Read the model definition and answer for the solid it produces. Units are mm, in the model's axes. Coordinates: 2 decimals unless noted, no trailing zeros. Write each loop counter-clockwise with the first axis right and the second up, starting at its lowest first coordinate (ties: lowest second). Pieces come first, ordered by that corner, then holes.
(1) Section A-A on x = 0.35 is taken. State how many separate pieces and enclosed holes the cut face has, then the cut area to 3 significant figures.
(2) Find the intervals of material crossed by probe 1 along Z at (x, y) = (0.4, 275); probe 2 along Y at (x, z) = (0.95, -1); probe 3 along Z at (x, y) = (0.7, 263.5), in increasing order.
(3) Section C-C on z = -7.5 is taken. Write down the section's boundary in (x, y).
(4) Given pin 1 (12 mm diameter, centred on y = 94.5, z = -6, fed in from -X); pin 2 (0.5 mm diameter, centred on x = 0.5, z = 15.5, fed in from +Y); pin 3 (0.5 mm diameter, centred on x = 0.5, z = 23, fed in from -Y), each flat-ended and moving along its own axis, determine where each tip first touches the part or whether it passes through.
from build123d import *

# Parameters (mm, degrees)
F1_DEPTH = 1


with BuildPart() as f1:
    # F0 (on Right) → F1 (new body)
    with BuildSketch(Plane.YZ):
        Polygon((289.166, 39.710689), (-29.834, 39.710689), (-56.334, 39.710689), (-56.334, 32.210689), (-29.834, 32.210689), (-29.834, -16.289311), (289.166, -16.289311), (289.166, 32.210689), (315.666, 32.210689), (315.666, 39.710689), align=None)
        with BuildLine():
            ThreePointArc((-24.167, 27.710689), (-23.581214, 29.124903), (-22.167, 29.710689))
            Line((-22.167, 29.710689), (-13.167, 29.710689))
            ThreePointArc((-13.167, 29.710689), (-11.752786, 29.124903), (-11.167, 27.710689))
            Line((-11.167, 27.710689), (-11.167, 10.710689))
            ThreePointArc((-11.167, 10.710689), (-11.752786, 9.296475), (-13.167, 8.710689))
            Line((-13.167, 8.710689), (-22.167, 8.710689))
            ThreePointArc((-22.167, 8.710689), (-23.581214, 9.296475), (-24.167, 10.710689))
            Line((-24.167, 10.710689), (-24.167, 27.710689))
        make_face(mode=Mode.SUBTRACT)
        with BuildLine():
            ThreePointArc((-5.5, 27.710689), (-4.914214, 29.124903), (-3.5, 29.710689))
            Line((-3.5, 29.710689), (19, 29.710689))
            ThreePointArc((19, 29.710689), (20.414214, 29.124903), (21, 27.710689))
            Line((21, 27.710689), (21, 10.710689))
            ThreePointArc((21, 10.710689), (20.414214, 9.296475), (19, 8.710689))
            Line((19, 8.710689), (-3.5, 8.710689))
            ThreePointArc((-3.5, 8.710689), (-4.914214, 9.296475), (-5.5, 10.710689))
            Line((-5.5, 10.710689), (-5.5, 27.710689))
        make_face(mode=Mode.SUBTRACT)
        with BuildLine():
            ThreePointArc((26.663, 27.710689), (27.248786, 29.124903), (28.663, 29.710689))
            Line((28.663, 29.710689), (51.163, 29.710689))
            ThreePointArc((51.163, 29.710689), (52.577214, 29.124903), (53.163, 27.710689))
            Line((53.163, 27.710689), (53.163, 10.710689))
            ThreePointArc((53.163, 10.710689), (52.577214, 9.296475), (51.163, 8.710689))
            Line((51.163, 8.710689), (28.663, 8.710689))
            ThreePointArc((28.663, 8.710689), (27.248786, 9.296475), (26.663, 10.710689))
            Line((26.663, 10.710689), (26.663, 27.710689))
        make_face(mode=Mode.SUBTRACT)
        with BuildLine():
            ThreePointArc((58.83, 27.710689), (59.415786, 29.124903), (60.83, 29.710689))
            Line((60.83, 29.710689), (83.33, 29.710689))
            ThreePointArc((83.33, 29.710689), (84.744214, 29.124903), (85.33, 27.710689))
            Line((85.33, 27.710689), (85.33, 10.710689))
            ThreePointArc((85.33, 10.710689), (84.744214, 9.296475), (83.33, 8.710689))
            Line((83.33, 8.710689), (60.83, 8.710689))
            ThreePointArc((60.83, 8.710689), (59.415786, 9.296475), (58.83, 10.710689))
            Line((58.83, 10.710689), (58.83, 27.710689))
        make_face(mode=Mode.SUBTRACT)
        with BuildLine():
            ThreePointArc((90.997, 27.710689), (91.582786, 29.124903), (92.997, 29.710689))
            Line((92.997, 29.710689), (115.497, 29.710689))
            ThreePointArc((115.497, 29.710689), (116.911214, 29.124903), (117.497, 27.710689))
            Line((117.497, 27.710689), (117.497, 10.710689))
            ThreePointArc((117.497, 10.710689), (116.911214, 9.296475), (115.497, 8.710689))
            Line((115.497, 8.710689), (92.997, 8.710689))
            ThreePointArc((92.997, 8.710689), (91.582786, 9.296475), (90.997, 10.710689))
            Line((90.997, 10.710689), (90.997, 27.710689))
        make_face(mode=Mode.SUBTRACT)
        with BuildLine():
            ThreePointArc((123.164, 27.710689), (123.749786, 29.124903), (125.164, 29.710689))
            Line((125.164, 29.710689), (147.664, 29.710689))
            ThreePointArc((147.664, 29.710689), (149.078214, 29.124903), (149.664, 27.710689))
            Line((149.664, 27.710689), (149.664, 10.710689))
            ThreePointArc((149.664, 10.710689), (149.078214, 9.296475), (147.664, 8.710689))
            Line((147.664, 8.710689), (125.164, 8.710689))
            ThreePointArc((125.164, 8.710689), (123.749786, 9.296475), (123.164, 10.710689))
            Line((123.164, 10.710689), (123.164, 27.710689))
        make_face(mode=Mode.SUBTRACT)
        with BuildLine():
            ThreePointArc((155.331, 27.710689), (155.916786, 29.124903), (157.331, 29.710689))
            Line((157.331, 29.710689), (179.831, 29.710689))
            ThreePointArc((179.831, 29.710689), (181.245214, 29.124903), (181.831, 27.710689))
            Line((181.831, 27.710689), (181.831, 10.710689))
            ThreePointArc((181.831, 10.710689), (181.245214, 9.296475), (179.831, 8.710689))
            Line((179.831, 8.710689), (157.331, 8.710689))
            ThreePointArc((157.331, 8.710689), (155.916786, 9.296475), (155.331, 10.710689))
            Line((155.331, 10.710689), (155.331, 27.710689))
        make_face(mode=Mode.SUBTRACT)
        with BuildLine():
            ThreePointArc((187.498, 27.710689), (188.083786, 29.124903), (189.498, 29.710689))
            Line((189.498, 29.710689), (211.998, 29.710689))
            ThreePointArc((211.998, 29.710689), (213.412214, 29.124903), (213.998, 27.710689))
            Line((213.998, 27.710689), (213.998, 10.710689))
            ThreePointArc((213.998, 10.710689), (213.412214, 9.296475), (211.998, 8.710689))
            Line((211.998, 8.710689), (189.498, 8.710689))
            ThreePointArc((189.498, 8.710689), (188.083786, 9.296475), (187.498, 10.710689))
            Line((187.498, 10.710689), (187.498, 27.710689))
        make_face(mode=Mode.SUBTRACT)
        with BuildLine():
            ThreePointArc((219.665, 27.710689), (220.250786, 29.124903), (221.665, 29.710689))
            Line((221.665, 29.710689), (244.165, 29.710689))
            ThreePointArc((244.165, 29.710689), (245.579214, 29.124903), (246.165, 27.710689))
            Line((246.165, 27.710689), (246.165, 10.710689))
            ThreePointArc((246.165, 10.710689), (245.579214, 9.296475), (244.165, 8.710689))
            Line((244.165, 8.710689), (221.665, 8.710689))
            ThreePointArc((221.665, 8.710689), (220.250786, 9.296475), (219.665, 10.710689))
            Line((219.665, 10.710689), (219.665, 27.710689))
        make_face(mode=Mode.SUBTRACT)
        with BuildLine():
            ThreePointArc((251.832, 27.710689), (252.417786, 29.124903), (253.832, 29.710689))
            Line((253.832, 29.710689), (262.832, 29.710689))
            ThreePointArc((262.832, 29.710689), (264.246214, 29.124903), (264.832, 27.710689))
            Line((264.832, 27.710689), (264.832, 10.710689))
            ThreePointArc((264.832, 10.710689), (264.246214, 9.296475), (262.832, 8.710689))
            Line((262.832, 8.710689), (253.832, 8.710689))
            ThreePointArc((253.832, 8.710689), (252.417786, 9.296475), (251.832, 10.710689))
            Line((251.832, 10.710689), (251.832, 27.710689))
        make_face(mode=Mode.SUBTRACT)
        with BuildLine():
            ThreePointArc((270.499, 27.710689), (271.084786, 29.124903), (272.499, 29.710689))
            Line((272.499, 29.710689), (281.499, 29.710689))
            ThreePointArc((281.499, 29.710689), (282.913214, 29.124903), (283.499, 27.710689))
            Line((283.499, 27.710689), (283.499, 10.710689))
            ThreePointArc((283.499, 10.710689), (282.913214, 9.296475), (281.499, 8.710689))
            Line((281.499, 8.710689), (272.499, 8.710689))
            ThreePointArc((272.499, 8.710689), (271.084786, 9.296475), (270.499, 10.710689))
            Line((270.499, 10.710689), (270.499, 27.710689))
        make_face(mode=Mode.SUBTRACT)
    extrude(amount=F1_DEPTH)


solid = f1.part
Response:
1. separate pieces: 1
1. enclosed holes: 11
1. area: 13,000 mm2
2. probe 1: z = -16.29 to 8.71, 29.71 to 39.71
2. probe 2: y = -29.83 to 289.17
2. probe 3: z = -16.29 to 8.83, 29.6 to 39.71
3. outline: (0, -29.83) - (1, -29.83) - (1, 289.17) - (0, 289.17) - close
4. pin 1: stops at x = 0
4. pin 2: stops at y = 289.17
4. pin 3: stops at y = -29.83
